from build123d import *

# Parameters (mm, degrees)
F0_W     = 25.4
F0_H     = 25.4
F1_DEPTH = 11.43
F2_W     = 10.16
F2_H     = 4.2333333333
F2_H_2   = 4.2418
F3_DEPTH = 2.54
F2_W_2   = 5.08
F4_DEPTH = 22.861
F5_R     = 1.27


with BuildPart() as f1:
    # F0 (on Top) → F1 (new body, symmetric)
    with BuildSketch(Plane.XY):
        Rectangle(F0_W, F0_H)
    extrude(amount=F1_DEPTH, both=True)

    # F2 (on face) → F3 (join)
    with BuildSketch(Plane.XY.offset(11.43)):
        Polygon((-2.54, 12.7), (-12.7, 12.7), (-12.7, -4.2333333333), (-8.4582, -4.2333333333), (-8.4582, 8.4666666667), (-2.54, 8.4666666667), align=None)
        with Locations((7.62, 10.5833333333)):
            Rectangle(F2_W, F2_H)
        Polygon((8.4666666667, -8.4582), (2.54, -8.4582), (2.54, -12.7), (12.7, -12.7), (12.7, 4.2333333333), (8.4666666667, 4.2333333333), align=None)
        Polygon((4.669733183, 0), (0, 4.669733183), (-4.669733183, 0), (0, -4.669733183), align=None)
        with Locations((-7.62, -10.5791)):
            Rectangle(F2_W, F2_H_2)
    extrude(amount=F3_DEPTH)

    # F2 (on face) → F4 (cut, through all)
    with BuildSketch(Plane.XY.offset(11.43)):
        with Locations((0, 10.5833333333)):
            Rectangle(F2_W_2, F2_H)
        with Locations((0, -10.5791)):
            Rectangle(F2_W_2, F2_H_2)
    extrude(amount=-F4_DEPTH, mode=Mode.SUBTRACT)

    # F5
    f5_edges = [f1.edges().sort_by_distance(p)[0] for p in [
        (-12.7, 12.7, 1.27),
        (-12.7, -12.7, 1.27),
        (12.7, 12.7, 1.27),
        (12.7, -12.7, 1.27),
        (2.54, -12.7, 1.27),
        (-2.54, -12.7, 1.27),
        (2.54, 12.7, 1.27),
        (-2.54, 12.7, 1.27),
    ]]
    fillet(f5_edges, radius=F5_R)


solid = f1.part
Here's how the part is built. I have some questions about the finished solid (model axes, mm). A direction names the side the tool comes from. Coordinates: 2 decimals unless noted, no trailing zeros. Loops run counter-clockwise (first coordinate to the right, second up) from the corner with the lowest first, then second, coordinate; pieces in that order, holes last. Notation, with made-up numbers: (66.25, 1.5) -> (70.25, 1.5) arc R23 cw to (70.25, 31.5) -> close; hole circle Ø2 at (-34.75, 38). An arc over 180 degrees is marked (long way). Use one line per item in the form item = value. Start each with the question number.
(1) If we section it at A-A (y = 9.5): Please give me the cut outline in (x, z), then the cut area to 3 significant figures.
(2) On a 3-axis mill with a long thin cutter (end or side, diameter ignored), from which of +Z, -Z, +X, -X, +Y, -Y can I reach the whole of each face in a straight line? I mean faces 5 (the face through (2.902, -12.318, 1.092)), 6 (the face through (0, 8.467, 0)), 7 (the face through (10, -6, 13.97)). Say none if no direction works.
(3) Will these pins go through, and if not, where does the flat tip stop? pin 1 (3 mm diameter, centred on x = 1, z = -7, fed in from +Y); pin 2 (1.5 mm diameter, centred on x = 1, z = 0, fed in from -Y).
(4) We'd pull the mould along Y, two halves only. Please class faces 1 (the face through (-6, 8.467, 13)), 2 (the face through (-11, -4.233, 13)), 3 (the face through (-2.922, -12.338, 1.092)), 4 (the face through (2.54, -10, 1)): pulls with the +Y half, pulls with the -Y half, needs draft (parallel to the pull), parting line crosses it, or undercut.
(5) If we section it at D-D (y = -0.5): Please give me the cut outline in (x, z).
(6) If we section it at B-B (x = 9.5): Please give me the cut outline in (y, z), then the cut area to 3 significant figures.
(7) If we section it at C-C (z = -9.5): Please give me the cut outline in (x, y), then the cut area to 3 significant figures.
(8) Please list where these lines run through material, in increasing order: line 1 along X through (y, z) = (-9.5, -2); line 2 along Y through (x, z) = (-2.5, 7.5); line 3 along Y through (x, z) = (10, 11.75).
Verdict:
q1.outline = (-12.7, -11.43) -> (-2.54, -11.43) -> (-2.54, 13.97) -> (-12.7, 13.97) -> close; (2.54, -11.43) -> (12.7, -11.43) -> (12.7, 13.97) -> (2.54, 13.97) -> close
q1.area = 516 mm²
q2.face_5 = +Z, -Z, -Y
q2.face_6 = +Z, -Z, +Y
q2.face_7 = +Z, +X, -X, +Y, -Y
q3.pin_1 = 8.47
q3.pin_2 = -8.46
q4.face_1 = undercut
q4.face_2 = undercut
q4.face_3 = pulls with the -Y half
q4.face_4 = needs draft
q5.outline = (-12.7, -11.43) -> (12.7, -11.43) -> (12.7, 13.97) -> (8.47, 13.97) -> (8.47, 11.43) -> (4.17, 11.43) -> (4.17, 13.97) -> (-4.17, 13.97) -> (-4.17, 11.43) -> (-8.46, 11.43) -> (-8.46, 13.97) -> (-12.7, 13.97) -> close
q6.outline = (-12.7, -11.43) -> (12.7, -11.43) -> (12.7, 13.97) -> (8.47, 13.97) -> (8.47, 11.43) -> (4.23, 11.43) -> (4.23, 13.97) -> (-12.7, 13.97) -> close
q6.area = 634 mm²
q7.outline = (-12.7, -11.43) arc R1.27 ccw to (-11.43, -12.7) -> (-3.81, -12.7) arc R1.27 ccw to (-2.54, -11.43) -> (-2.54, -8.46) -> (2.54, -8.46) -> (2.54, -11.43) arc R1.27 ccw to (3.81, -12.7) -> (11.43, -12.7) arc R1.27 ccw to (12.7, -11.43) -> (12.7, 11.43) arc R1.27 ccw to (11.43, 12.7) -> (3.81, 12.7) arc R1.27 ccw to (2.54, 11.43) -> (2.54, 8.47) -> (-2.54, 8.47) -> (-2.54, 11.43) arc R1.27 ccw to (-3.81, 12.7) -> (-11.43, 12.7) arc R1.27 ccw to (-12.7, 11.43) -> close
q7.area = 599 mm²
q8.line_1 = -12.7 to -2.54, 2.54 to 12.7
q8.line_2 = -8.46 to 8.47
q8.line_3 = -12.7 to 4.23, 8.47 to 12.7
